Source: three-view drawing plus pictorial views. Frame: mm from the lowest corner of the part. A direction names the side the tool comes from. Round coordinates to 2 decimals unless told otherwise and drop trailing zeros. Loops run counter-clockwise (first coordinate to the right, second up) from the corner with the lowest first, then second, coordinate; pieces in that order, holes last. Notation, with made-up numbers: (68, 1) -> (124, 1) arc R30 cw to (124, 38) -> close; hole circle Ø10 at (69, 82.5). An arc over 180 degrees is marked (long way). Put each result on its own line as item: value. Start each with the question number.
1. Cut plane D-D (x = 18.5). Return the cut outline in (y, z) (1 decimal).
2. Material intervals for L1, parallel to Z at x = 17.5, y = 2.75 (1 decimal); L2, parallel to Z at x = 2.75, y = 10.5 (1 decimal); L3, parallel to Y at x = 18.5, z = 9.5 (1 decimal), sorted ascending.
3. Draft query along X for the marked faces 5, 6 and 7. Return one class per face: pulls with the +X half, pulls with the -X half, needs draft (parallel to the pull), parting line crosses it, or undercut.
4. Cut plane C-C (x = 13.25). Return the cut outline in (y, z) (1 decimal), then the cut area to 3 significant figures.
5. Set-up query: the marked faces 1, 2, 3 and 4. Return all of +Z, -Z, +X, -X, +Y, -Y with unobstructed straight access to the full face (end or side cutting, diameter ignored); none if empty.
6. Cut plane A-A (y = 10.25). Return the cut outline in (x, z) (1 decimal).
7. Contact query for flat-ended pins moving along their axis: pin 1 (2.5 mm diameter, centred on x = 27, y = 11.5, fed in from +Z); pin 2 (3.5 mm diameter, centred on x = 11, z = 8.5, fed in from -Y); pin 3 (1.1 mm diameter, centred on x = 27.5, y = 11, fed in from -Z) (1 decimal). Output: stop coordinate, or through.
8. Cut plane B-B (z = 7.75). Return the cut outline in (x, y) (1 decimal), then the cut area to 3 significant figures.
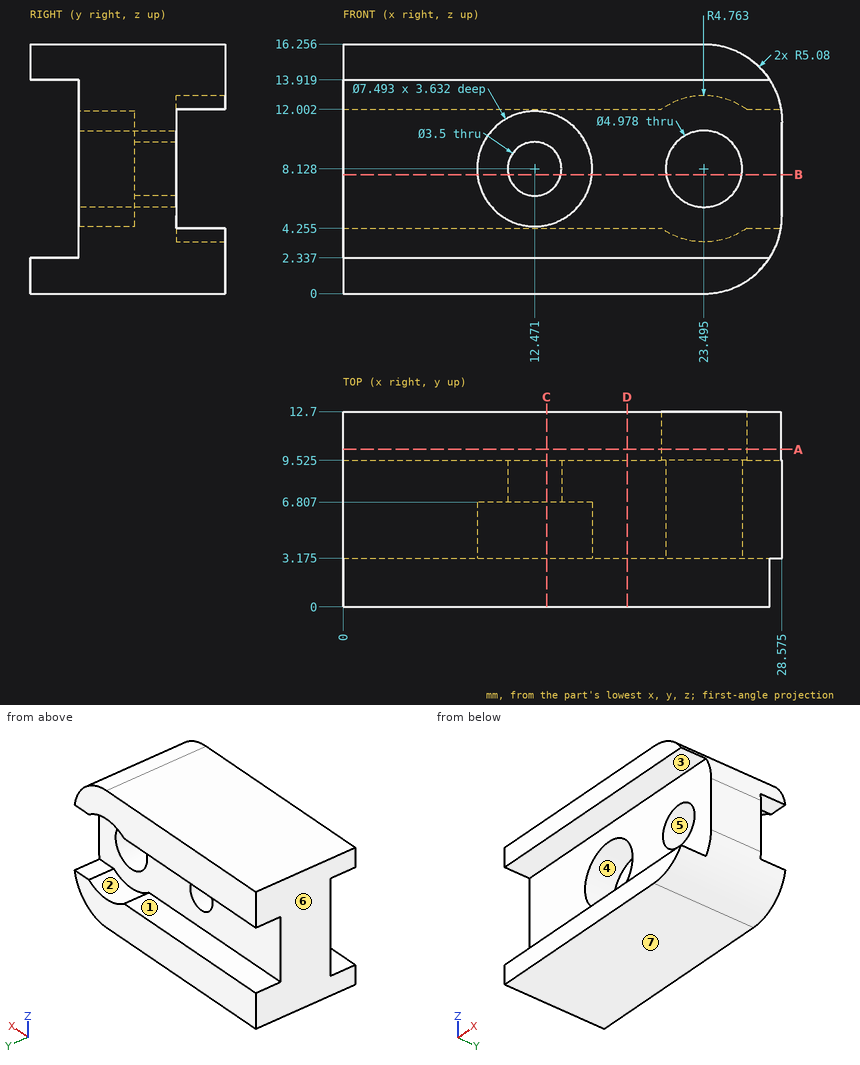
Solution:
1. outline: (0, 0) -> (12.7, 0) -> (12.7, 4.3) -> (9.5, 4.3) -> (9.5, 12) -> (12.7, 12) -> (12.7, 16.3) -> (0, 16.3) -> (0, 13.9) -> (3.2, 13.9) -> (3.2, 2.3) -> (0, 2.3) -> close
2. L1: z = 0 to 2.3, 13.9 to 16.3
2. L2: z = 0 to 4.3, 12 to 16.3
2. L3: y = 3.2 to 9.5
3. face 5: undercut
3. face 6: pulls with the -X half
3. face 7: needs draft
4. outline: (0, 0) -> (12.7, 0) -> (12.7, 4.3) -> (9.5, 4.3) -> (9.5, 6.6) -> (6.8, 6.6) -> (6.8, 4.5) -> (3.2, 4.5) -> (3.2, 2.3) -> (0, 2.3) -> close; (0, 13.9) -> (3.2, 13.9) -> (3.2, 11.8) -> (6.8, 11.8) -> (6.8, 9.7) -> (9.5, 9.7) -> (9.5, 12) -> (12.7, 12) -> (12.7, 16.3) -> (0, 16.3) -> close
4. area: 110 mm^2
5. face 1: +X, -X, +Y
5. face 2: +Y
5. face 3: +X, -X, -Y
5. face 4: -Y
6. outline: (0, 0) -> (23.5, 0) arc R5.1 ccw to (28.5, 4.3) -> (26.3, 4.3) arc R4.8 cw to (20.7, 4.3) -> (0, 4.3) -> close; (0, 12) -> (20.7, 12) arc R4.8 cw to (26.3, 12) -> (28.5, 12) arc R5.1 ccw to (23.5, 16.3) -> (0, 16.3) -> close
7. pin 1: stops at z = 15.73
7. pin 2: stops at y = 6.81
7. pin 3: stops at z = 1.4
8. outline: (0, 3.2) -> (8.7, 3.2) -> (8.7, 6.8) -> (10.8, 6.8) -> (10.8, 9.5) -> (0, 9.5) -> close; (14.2, 6.8) -> (16.2, 6.8) -> (16.2, 3.2) -> (21, 3.2) -> (21, 9.5) -> (14.2, 9.5) -> close; (26, 3.2) -> (28.6, 3.2) -> (28.6, 9.5) -> (26, 9.5) -> close
8. area: 114 mm^2
